Check sheet for the drawn part. Datum: minimum x, y, z corner. Units: mm. Coordinates: 2 decimals unless noted, no trailing zeros. Write each loop counter-clockwise with the first axis right and the second up, starting at its lowest first coordinate (ties: lowest second). Pieces come first, ordered by that corner, then holes. Notation, with made-up numbers: M -30,34 L 28,34 A25 ccw 28,55 Z; hole C 80,80.25 d9. An arc over 180 degrees is marked long. Answer as CSV lines item,"result".
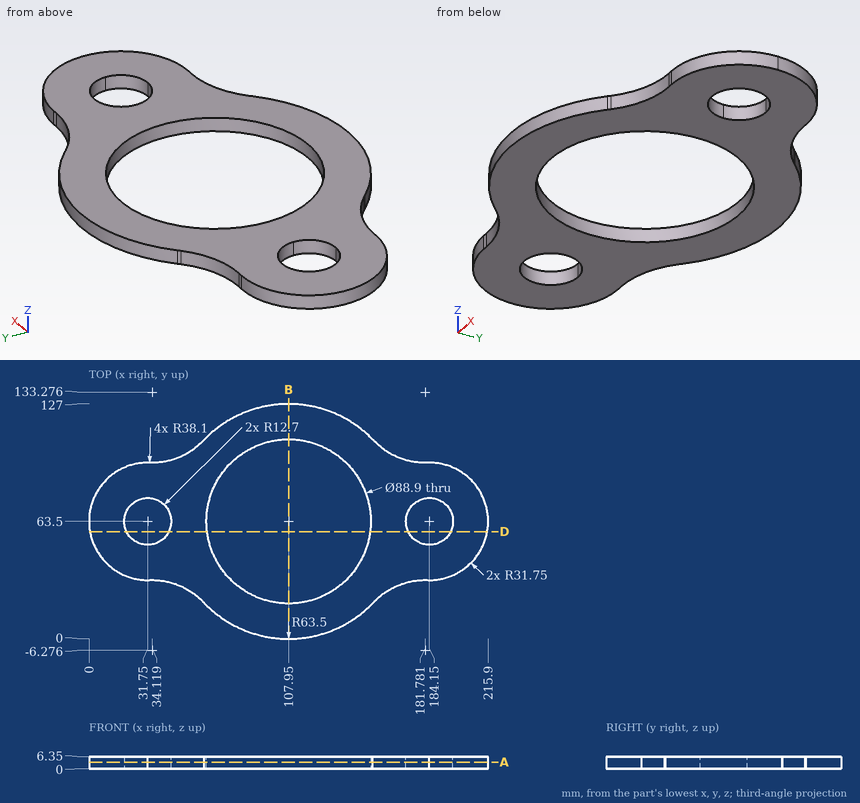
1) Thickness scan on line 1 along X through (y, z) = (83, 4) (1 decimal); line 2 along X through (y, z) = (54.5, 6); line 3 along X through (y, z) = (29, 2.25) (1 decimal). Record the ranges inside material, lowest first.
Answer key:
line 1,"x = 6.7 to 68, 147.9 to 209.2"
line 2,"x = 1.3 to 22.79, 40.71 to 64.42, 151.48 to 175.19, 193.11 to 214.6"
line 3,"x = 48.5 to 79.9, 136 to 167.4"
2) Section check A-A, the plane z = 3.5. Record the boundary of the cut face in (x, y), plus the area to 3 significant figures.
Answer key:
outline,"M 31.75,31.75 A38.1 cw 62.36,19.3 A63.5 ccw 153.54,19.3 A38.1 cw 184.15,31.75 A31.75 ccw 184.15,95.25 A38.1 cw 153.54,107.7 A63.5 ccw 62.36,107.7 A38.1 cw 31.75,95.25 A31.75 ccw Z; hole C 31.75,63.5 d25.4; hole C 107.95,63.5 d88.9; hole C 184.15,63.5 d25.4"
area,"10,700 mm2"
3) Depth check by flat-ended pin: P1, Ø1, axis at x = 58.5, z = 3, coming from the +Y side; P2, Ø10, axis at x = 144.5, y = 105.5, coming from the -Z side; P3, Ø3, axis at x = 141, z = 4, coming from the +Y side. Enter the tip coordinate at first touch or a pass-through.
Answer key:
P1,"stops at y = 104.42"
P2,"stops at z = 0"
P3,"stops at y = 118.61"
4) Section check B-B, the plane x = 107.95. Record the boundary of the cut face in (y, z), plus the area to 3 significant figures.
Answer key:
outline,"M 0,0 L 19.05,0 L 19.05,6.35 L 0,6.35 Z; M 107.95,0 L 127,0 L 127,6.35 L 107.95,6.35 Z"
area,"242 mm2"
5) Section check D-D, the plane y = 58. Record the boundary of the cut face in (x, z), plus the area to 3 significant figures.
Answer key:
outline,"M 0.48,0 L 20.3,0 L 20.3,6.35 L 0.48,6.35 Z; M 43.2,0 L 63.84,0 L 63.84,6.35 L 43.2,6.35 Z; M 152.06,0 L 172.7,0 L 172.7,6.35 L 152.06,6.35 Z; M 195.6,0 L 215.42,0 L 215.42,6.35 L 195.6,6.35 Z"
area,"514 mm2"
